```python
from build123d import *

# Parameters (mm, degrees)
BOSS_EXTRUDE1_DEPTH = 75
SHELL1_START        = 1
SHELL1_DEPTH        = 73


# Read off the part's stored shape, not the designer's step: Shell1
with BuildPart() as part:
    # Sketch2 → Boss-Extrude1 (new body)
    with BuildSketch(Plane(origin=(0, 0, 0), x_dir=(0, 0, -1), z_dir=(1, 0, 0))):
        with BuildLine():
            Line((-10.5, -9), (10.5, -9))
            Line((10.5, -9), (10.5, 6))
            ThreePointArc((10.5, 6), (9.621320344, 8.121320344), (7.5, 9))
            Line((7.5, 9), (-7.5, 9))
            ThreePointArc((-7.5, 9), (-9.621320344, 8.121320344), (-10.5, 6))
            Line((-10.5, 6), (-10.5, -9))
        make_face()
    extrude(amount=BOSS_EXTRUDE1_DEPTH)

    # Shell1 outline → Shell1 (cut)
    with BuildSketch(Plane.YZ.offset(SHELL1_START)):
        with BuildLine():
            Line((8, -7.5), (9, -7.5))
            Line((9, -7.5), (9, 7.5))
            Line((9, 7.5), (8, 7.5))
            ThreePointArc((8, 7.5), (7.414213562, 8.914213562), (6, 9.5))
            Line((6, 9.5), (-8, 9.5))
            Line((-8, 9.5), (-8, -9.5))
            Line((-8, -9.5), (6, -9.5))
            ThreePointArc((6, -9.5), (7.414213562, -8.914213562), (8, -7.5))
        make_face()
    extrude(amount=SHELL1_DEPTH, mode=Mode.SUBTRACT)


solid = part.part
```
Build history of the part. All positions in model axes, mm. A direction names the side the tool comes from. Give positions to 0.01 mm unless a question says otherwise; leave off trailing zeros. Loops run counter-clockwise (first coordinate to the right, second up) from the corner with the lowest first, then second, coordinate; pieces in that order, holes last.
Item 1: Slice it at B-B, the plane x = 42. List the corners of the cut face in (y, z).
Answers follow:
outline: (-9, -10.5) - (6, -10.5) arc R3 ccw to (9, -7.5) - (8, -7.5) arc R2 cw to (6, -9.5) - (-8, -9.5) - (-8, 9.5) - (6, 9.5) arc R2 cw to (8, 7.5) - (9, 7.5) arc R3 ccw to (6, 10.5) - (-9, 10.5) - close
Item 2: Slice it at C-C, the plane z = 6.5. List the corners of the cut face in (x, y).
Answers follow:
outline: (0, -9) - (75, -9) - (75, 9) - (74, 9) - (74, -8) - (1, -8) - (1, 9) - (0, 9) - close
Item 3: Drill centre lines: line 1 (X direction, y = -7.5, z = -2.5); line 2 (Z direction, x = 55, y = -0.75); line 3 (Y direction, x = 37.5, z = -4). Where is each one in solid material? Low to high.
Answers follow:
line 1: x = 0 to 1, 74 to 75
line 2: z = -10.5 to -9.5, 9.5 to 10.5
line 3: y = -9 to -8
Item 4: Slice it at A-A, the plane y = 1.5. List the corners of the cut face in (x, z).
Answers follow:
outline: (0, -10.5) - (75, -10.5) - (75, 10.5) - (0, 10.5) - close; hole (1, -9.5) - (74, -9.5) - (74, 9.5) - (1, 9.5) - close
Item 5: Which spindle directions (+Z, -Z, +X, -X, +Y, -Y) get a long thin tool onto all of the face, cutting with end or side? Do faces 5 (the face through (37, -9, 0)), 6 (the face through (37, -1, 9.5)). Say none if no direction does.
Answers follow:
face 5: +Z, -Z, +X, -X, -Y
face 6: none
Item 6: Pull direction Z, two halves, no side cores. Call faces 1 (the face through (36.98, 8.14, 9.6)), 2 (the face through (36.99, 7.43, 8.9)), 3 (the face through (0, 0, 0)), 4 (the face through (36.98, 8.1, -9.64)): released by +Z, released by -Z, zero draft, split by the parting line, or undercut.
Answers follow:
face 1: released by +Z
face 2: undercut
face 3: zero draft
face 4: released by -Z
Item 7: Flat gauge pins, fed straight in: pin 1 (1 mm diameter, centred on y = 2, z = -4.5, fed in from -X); pin 2 (0.8 mm diameter, centred on x = 44, y = 8.5, fed in from -Z). Where does each tip first touch, or does it go through?
Answers follow:
pin 1: stops at x = 0
pin 2: stops at z = -9.64
